Autodesk Inventor part; units mm, degrees
ref_plane "YZ Plane" through (0, 0, 0) normal (1, 0, 0) x (0, 1, 0)
ref_plane "XZ Plane" through (0, 0, 0) normal (0, 1, 0) x (-1, 0, 0)
ref_plane "XY Plane" through (0, 0, 0) normal (0, 0, 1) x (1, 0, 0)
sketch "Sketch1" plane through (0, 0, 0) normal (0, 1, 0) x (-1, 0, 0)
  line L0 (-9.525, -8.255) -> (9.525, -8.255)
  line L1 (9.525, -8.255) -> (9.525, 8.255)
  line L2 (9.525, 8.255) -> (-9.525, 8.255)
  line L3 (-9.525, 8.255) -> (-9.525, -8.255)
  line L4 (-9.525, -8.255) -> (9.525, 8.255) construction
  line L5 (9.525, -8.255) -> (-9.525, 8.255) construction
  point P0 (0, 0)
  dimension "d9" = 19.05
  dimension "d10" = 16.51
extrude "Extrusion3" add sketch "Sketch1" along normal blind 25.4
sketch "actual_circle" plane through (0, 25.4, 0) normal (0, 1, 0) x (1, 0, 0)
  circle A0 centre (0, 0) radius 5.5563
  dimension "d27" = 11.1125
extrude "Extrusion6" cut sketch "actual_circle" against normal blind 50.8
sketch "circle" plane through (-9.525, 0, 8.255) normal (0, 0, 1) x (1, 0, 0)
  line L0 (2.54, 20.32) -> (16.51, 20.32)
  line L1 (16.51, 20.32) -> (16.51, 5.08)
  line L2 (16.51, 5.08) -> (2.54, 5.08)
  line L3 (2.54, 5.08) -> (2.54, 20.32)
  line L4 (0, 25.4) -> (19.05, 25.4)
  line L5 (0, 0) -> (0, 25.4)
  point P0 (9.525, 0)
  dimension "d32" = 13.97
  dimension "d33" = 15.24
  dimension "d34" = 5.08
  dimension "d35" = 2.54
extrude "Extrusion7" cut sketch "circle" against normal blind 2.286
sketch "Sketch7" plane through (9.525, 0, -8.255) normal (0, 0, -1) x (-1, 0, 0)
  line L0 (2.54, 20.32) -> (16.51, 20.32)
  line L1 (16.51, 20.32) -> (16.51, 5.08)
  line L2 (16.51, 5.08) -> (2.54, 5.08)
  line L3 (2.54, 5.08) -> (2.54, 20.32)
  line L4 (0, 0) -> (0, 25.4)
  line L5 (0, 25.4) -> (19.05, 25.4)
  point P0 (9.525, 0)
  dimension "d38" = 13.97
  dimension "d39" = 15.24
  dimension "d40" = 2.54
  dimension "d41" = 5.08
extrude "Extrusion8" cut sketch "Sketch7" against normal blind 2.286
sketch "Lock" plane through (-6.985, 5.08, -8.255) normal (1, 0, 0) x (0, 0, -1)
  line L0 (-0.762, 7.874) -> (0, 7.874)
  line L1 (0, 7.874) -> (0, 4.826)
  line L2 (0, 4.826) -> (-0.762, 4.826)
  line L3 (-0.762, 4.826) -> (-0.762, 7.874)
  line L4 (-2.286, 15.24) -> (-2.286, 0)
  point P0 (-8.255, -5.08)
  point P1 (0, 15.24)
  dimension "d44" = 0.762
  dimension "d45" = 3.048
  dimension "d46" = 7.366
  dimension "d47" = 1.524
extrude "Extrusion9" add sketch "Lock" along normal blind 13.97
sketch "Sketch9" plane through (-6.985, 5.08, 8.255) normal (1, 0, 0) x (0, 0, -1)
  line L0 (0, 7.874) -> (0.762, 7.874)
  line L1 (0.762, 7.874) -> (0.762, 4.826)
  line L2 (0.762, 4.826) -> (0, 4.826)
  line L3 (0, 4.826) -> (0, 7.874)
  line L4 (0, 0) -> (0, 15.24)
  point P0 (8.255, -5.08)
  dimension "d50" = 0.762
  dimension "d51" = 3.048
  dimension "d52" = 0
  dimension "d53" = 7.366
extrude "Extrusion10" add sketch "Sketch9" along normal blind 13.97
fillet "Fillet1" radius 3.175 4 edges at (-9.525, 25.4, 0) (9.525, 25.4, 0) (0, 25.4, 8.255) (0, 25.4, -8.255)
properties part number "Weird_Box_Lina_Made_Me_Make_Final"
Check sheet for the modelled part. Datum: model origin and axes. Units: mm. A direction names the side the tool comes from. Give positions to 0.01 mm unless a question says otherwise; leave off trailing zeros. Loops run counter-clockwise (first coordinate to the right, second up) from the corner with the lowest first, then second, coordinate; pieces in that order, holes last. Notation, with made-up numbers: M 82,63.5 L 100,63.5 A19 cw 100,91.5 Z; hole C -24,-11.75 d6. An arc over 180 degrees is marked long. Answer as a JSON object with one key per item and string values. Group by question number.
Q1. Cross-section at B-B on z = 0. Record the cut outline in (x, y) (3 decimals).
Q2. Cross-section at C-C on y = 7. Record the cut outline in (x, z) (3 decimals), then the cut area to 3 significant figures.
Q3. Go/stop test with a flat-tipped pin: P1, Ø2.5, axis at x = 2, z = 7.5, coming from the +Y side. Record where the tip stops, or that it passes through.
Q4. Release check for a two-part mould opening along Y. For faces 1 (the cylindrical face through (-5.131, 24.495, -7.3)), 2 (the flat face through (0, 20.32, -7)), 3 (the cylindrical face through (-1.204, 12.878, 5.424)) record: released by +Y, released by -Y, zero draft, split by the parting line, or undercut.
Q5. Access from +Z, -Z, +X, -X, +Y, -Y to the whole of each face (thin tool, end or side, straight path). Record for faces 4 (the flat face through (0, 5.08, -7)), 5 (the flat face through (0, 20.32, 7)), 6 (the cylindrical face through (-5.029, 24.495, 7.3)), 7 (the flat face through (-6.985, 13, 7)), 8 (the cylindrical face through (5.029, 24.495, -7.3)).
Q6. Cross-section at A-A on y = 11. Record the cut outline in (x, z) (3 decimals), then the cut area to 3 significant figures.
Q7. Cross-section at D-D on x = 0. Give the number of separate pieces and of enclosed holes in the cut face, then the cut area to 3 significant figures.
Q8. Material ranges on line 1 along Z through (x, y) = (0, 10) (3 decimals); line 2 along X through (y, z) = (12.5, 0) (3 decimals); line 3 along Z through (x, y) = (0, 6), recorded low to high. Write a range as [from, to].
Evaluation:
{
 "1": {"outline": "M -9.525,0 L -5.556,0 L -5.556,25.4 L -6.35,25.4 A3.175 ccw -9.525,22.225 Z; M 5.556,0 L 9.525,0 L 9.525,22.225 A3.175 ccw 6.35,25.4 L 5.556,25.4 Z"},
 "2": {"outline": "M -9.525,-8.255 L -6.985,-8.255 L -6.985,-5.969 L 6.985,-5.969 L 6.985,-8.255 L 9.525,-8.255 L 9.525,8.255 L 6.985,8.255 L 6.985,5.969 L -6.985,5.969 L -6.985,8.255 L -9.525,8.255 Z; hole C 0,0 d11.113", "area": "154 mm2"},
 "3": {"P1": "stops at y = 25.18"},
 "4": {"face 1": "released by +Y", "face 2": "undercut", "face 3": "zero draft"},
 "5": {"face 4": "-Z", "face 5": "+Z", "face 6": "+Z, -X, +Y", "face 7": "none", "face 8": "-Z, +X, +Y"},
 "6": {"outline": "M -9.525,-8.255 L 9.525,-8.255 L 9.525,8.255 L -9.525,8.255 Z; hole M -6.985,-7.493 L 6.985,-7.493 L 6.985,-5.969 L -6.985,-5.969 Z; hole M -6.985,5.969 L 6.985,5.969 L 6.985,7.493 L -6.985,7.493 Z; hole C 0,0 d11.113", "area": "175 mm2"},
 "7": {"separate pieces": "4", "enclosed holes": "0", "area": "67.9 mm2"},
 "8": {"line 1": "z = [-8.255, -7.493], [-5.969, -5.556], [5.556, 5.969], [7.493, 8.255]", "line 2": "x = [-9.525, -5.556], [5.556, 9.525]", "line 3": "z = [-5.97, -5.56], [5.56, 5.97]"}
}
